Autodesk Inventor part; units mm, degrees
ref_plane "YZ Plane" through (0, 0, 0) normal (1, 0, 0) x (0, 1, 0)
ref_plane "XZ Plane" through (0, 0, 0) normal (0, 1, 0) x (-1, 0, 0)
ref_plane "XY Plane" through (0, 0, 0) normal (0, 0, 1) x (1, 0, 0)
sketch "Sketch1" plane through (0, 0, 0) normal (0, 1, 0) x (-1, 0, 0)
  line L0 (10, -45) -> (-10, -45)
  line L1 (-10, -45) -> (-10, 45)
  line L2 (-10, 45) -> (10, 45)
  line L3 (10, 45) -> (10, -45)
  point P0 (0, 0)
  dimension "d0" = 20
  dimension "d1" = 90
  dimension "d2" = 45
  dimension "d3" = 10
extrude "Plate1" add sketch "Sketch1" along normal blind 1.5
sketch "Sketch2" plane through (0, 0, 0) normal (0, -1, 0) x (1, 0, 0)
  circle A0 centre (0, 42) radius 0.7835
  circle A1 centre (-7, 35) radius 0.7835
  circle A2 centre (0, 28) radius 0.7835
  circle A3 centre (7, 35) radius 0.7835
  circle A4 centre (0, -28) radius 0.7835
  circle A5 centre (-7, -35) radius 0.7835
  circle A6 centre (0, -42) radius 0.7835
  circle A7 centre (7, -35) radius 0.7835
  point P0 (0, 0)
hole "Hole1" at (0, 0, 42) at (-7, 0, 35) at (0, 0, 28) at (7, 0, 35) at (0, 0, -28) at (-7, 0, -35) at (0, 0, -42) at (7, 0, -35) direction (0, 1, 0) diameter 2.1 depth 1.5
sketch "Sketch3" plane through (0, 1.5, 0) normal (0, 1, 0) x (1, 0, 0)
  arc A0 (10, 35) -> (-10, 35) centre (0, 35) ccw
  arc A1 (-10, -35) -> (10, -35) centre (0, -35) ccw
  line L0 (-10, 35) -> (-10, -35)
  line L1 (10, 35) -> (10, -35)
  line L2 (10, 45) -> (10, -45)
  line L3 (-10, 45) -> (10, 45)
  line L4 (10, 45) -> (10, -45)
  line L5 (10, -45) -> (-10, -45)
  line L6 (-10, -45) -> (-10, 45)
  point P0 (0, 0)
  point P1 (0, 45)
  point P2 (10, 35)
  point P3 (-10, -35)
  point P4 (0, -45)
  point P5 (10, -35)
  dimension "d12" = 35
  dimension "d13" = 35
  dimension "d14" = 10
  dimension "d15" = 10
  dimension "d16" = 10
  dimension "d17" = 20
  dimension "d18" = 90
extrude "Extrusion1" cut sketch "Sketch3" against normal blind 10 contours A0 L3 L2 | A0 L6 L3 | L2 L5 A1 | L5 L6 A1
sketch "Sketch4" plane through (0, 1.5, 0) normal (0, 1, 0) x (1, 0, 0)
  arc A0 (10, 35) -> (-10, 35) centre (0, 35) ccw
  arc A1 (-10, -35) -> (10, -35) centre (0, -35) ccw
  point P0 (0, 0)
hole "Hole2" at (0, 1.5, -35) at (0, 1.5, 35) direction (0, -1, 0) diameter 5.2 depth 1.5
equation "\"d10\" = Thickness"
equation "\"d26\" = Thickness"
equation "\"d4\" = Thickness"
equation "\"BendReliefWidth\" = Thickness"
equation "\"BendReliefDepth\" = 0.5 * Thickness"
equation "\"CornerReliefSize\" = 4 * Thickness"
equation "\"MinimumRemnant\" = 2 * Thickness"
equation "\"TransitionRadius\" = BendRadius"
equation "\"JacobiRadiusSize\" = BendRadius"
equation "\"GapSize\" = Thickness"
properties part number "axis_10_11-connector_frame" material "Aluminum 6061-AHC"
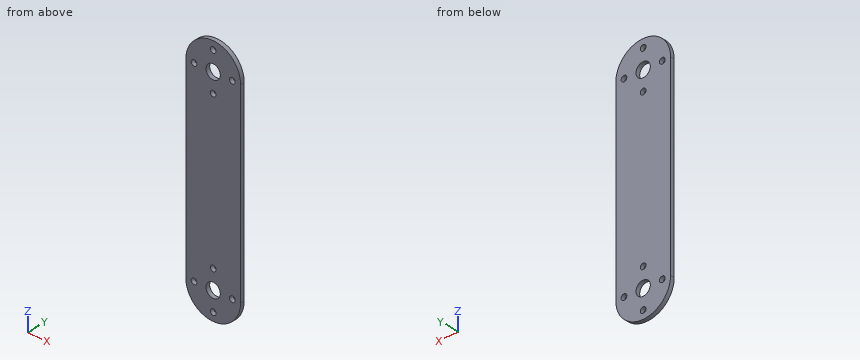
Model file for the job. Use its own axes, mm. Coordinates: 2 decimals unless noted, no trailing zeros. Loops run counter-clockwise (first coordinate to the right, second up) from the corner with the lowest first, then second, coordinate; pieces in that order, holes last. Notation, with made-up numbers: (5.25, -11.5) -> (58.25, -11.5) arc R20 cw to (58.25, 1.5) -> close; hole circle Ø11 at (32, 55). An arc over 180 degrees is marked (long way). Use one line per item in the form item = value. Start each with the question number.
(1) Cut at A-A on x = 0. Give the cut face in (y, z), and give its area (3 significant figures).
(2) Flat gauge pin, fed straight in: pin 1 (6 mm diameter, centred on x = -0.5, z = 20, fed in from -Y). Where does the tip first touch, or does it go through?
(3) Cut at B-B on z = 28. Give the cut face in (x, y), and give its area (4 significant figures).
(4) Cut at D-D on x = -7. Give the cut face in (y, z).
(5) Probe probe 1 along X at (y, z) = (0.35, 35); probe 2 along Z at (x, y) = (7, 0.7); probe 3 along X at (y, z) = (0.9, 42). List the from-to ranges inside material, lowest first. Write a range as from..to.
(6) Cut at C-C on y = 0.25. Give the number of separate pieces and of enclosed holes in the cut face, and give its area (3 significant figures).
Values:
q1.outline = (0, -45) -> (1.5, -45) -> (1.5, -43.05) -> (0, -43.05) -> close; (0, -40.95) -> (1.5, -40.95) -> (1.5, -37.6) -> (0, -37.6) -> close; (0, -32.4) -> (1.5, -32.4) -> (1.5, -29.05) -> (0, -29.05) -> close; (0, -26.95) -> (1.5, -26.95) -> (1.5, 26.95) -> (0, 26.95) -> close; (0, 29.05) -> (1.5, 29.05) -> (1.5, 32.4) -> (0, 32.4) -> close; (0, 37.6) -> (1.5, 37.6) -> (1.5, 40.95) -> (0, 40.95) -> close; (0, 43.05) -> (1.5, 43.05) -> (1.5, 45) -> (0, 45) -> close
q1.area = 107 mm2
q2.pin_1 = 0
q3.outline = (-10, 0) -> (-1.05, 0) -> (-1.05, 1.5) -> (-10, 1.5) -> close; (1.05, 0) -> (10, 0) -> (10, 1.5) -> (1.05, 1.5) -> close
q3.area = 26.85 mm2
q4.outline = (0, -42.14) -> (1.5, -42.14) -> (1.5, -36.05) -> (0, -36.05) -> close; (0, -33.95) -> (1.5, -33.95) -> (1.5, 33.95) -> (0, 33.95) -> close; (0, 36.05) -> (1.5, 36.05) -> (1.5, 42.14) -> (0, 42.14) -> close
q5.probe_1 = -10..-8.05, -5.95..-2.6, 2.6..5.95, 8.05..10
q5.probe_2 = -42.14..-36.05, -33.95..33.95, 36.05..42.14
q5.probe_3 = -7.14..-1.05, 1.05..7.14
q6.separate_pieces = 1
q6.enclosed_holes = 10
q6.area = 1,640 mm2
